Check sheet for the modelled part. Datum: model origin and axes. Units: mm. Face numbers are marked on the shaded views. A direction names the side the tool comes from. Coordinates: 2 decimals unless noted, no trailing zeros. Loops run counter-clockwise (first coordinate to the right, second up) from the corner with the lowest first, then second, coordinate; pieces in that order, holes last. Notation, with made-up numbers: (13.25, 64) -> (67.25, 64) arc R28 cw to (67.25, 89) -> close; hole circle Ø7 at (26.5, -6). An arc over 180 degrees is marked (long way). Use CSV: the item, a comma, the result in double quotes. Start each with the question number.
1. Sectioned sample at D-D, the plane x = 16.25. Record the cut outline in (y, z), and give its area (3 significant figures).
2. Sectioned sample at B-B, the plane z = 12.4. Record the cut outline in (x, y) (3 decimals), and give its area (3 significant figures).
3. Set-up check for the marked faces 4, 5, 6, 7 and 8: record each of +Z, -Z, +X, -X, +Y, -Y from which the full face is reachable in a straight line by a thin tool's end or side.
4. Release check for a two-part mould opening along Z. For the marked faces 1, 2 and 3 record: pulls with the +Z half, pulls with the -Z half, needs draft (parallel to the pull), parting line crosses it, or undercut.
5. Sectioned sample at C-C, the plane z = 4. Record the cut outline in (x, y) (3 decimals).
6. Thickness scan on L1, parallel to X at y = 0.6, z = 12.4; L2, parallel to Z at x = -16.25, y = 8.25; L3, parallel to Z at x = 10.5, y = 4.25 (3 decimals). Record the ranges inside material, lowest first.
7. Gauge pin test, flat ends, axial feed: pin 1 (1 mm diameter, centred on y = 9.5, z = 14, fed in from +X); pin 2 (2 mm diameter, centred on x = 16, z = 17, fed in from -Y); pin 3 (2 mm diameter, centred on x = 2, z = -13, fed in from +Y). Record the tip position at first contact, or that the pin passes through.
8. Sectioned sample at A-A, the plane y = 7. Record the cut outline in (x, z).
```python
from build123d import *

# Parameters (mm, degrees)
SKETCH1_W                      = 40
SKETCH1_H                      = 40
BOSS_EXTRUDE1_DEPTH            = 6.35
SKETCH2_W                      = 11.25
SKETCH2_H                      = 11.25
CUT_EXTRUDE1_DEPTH             = 7.35
SKETCH3_W                      = 14
SKETCH3_H                      = 8.5
CUT_EXTRUDE2_DEPTH             = 2
M2_CLEARANCE_HOLE1_D           = 2.4
SKETCH6_R                      = 2.6
BOSS_EXTRUDE2_DEPTH            = 5
CBORE_FOR_M2_SHCS1_D           = 2.4
CBORE_FOR_M2_SHCS1_CBORE_D     = 4.4
CBORE_FOR_M2_SHCS1_CBORE_DEPTH = 2
SKETCH13_R                     = 2.175
CUT_EXTRUDE4_DEPTH             = 4.2
CHAMFER1_SIZE                  = 2.5


with BuildPart() as part:
    # Sketch1 → Boss-Extrude1 (new body)
    with BuildSketch(Plane(origin=(0, 0, 0), x_dir=(1, 0, 0), z_dir=(0, 1, 0))):
        Rectangle(SKETCH1_W, SKETCH1_H)
    extrude(amount=BOSS_EXTRUDE1_DEPTH)

    # Sketch2 → Cut-Extrude1 (cut, through all)
    with BuildSketch(Plane(origin=(0, 6.35, 0), x_dir=(1, 0, 0), z_dir=(0, 1, 0))):
        Rectangle(SKETCH2_W, SKETCH2_H)
    extrude(amount=-CUT_EXTRUDE1_DEPTH, mode=Mode.SUBTRACT)

    # Sketch3 → Cut-Extrude2 (cut)
    with BuildSketch(Plane(origin=(0, 6.35, 0), x_dir=(1, 0, 0), z_dir=(0, 1, 0))):
        with Locations((0, -9.875)):
            Rectangle(SKETCH3_W, SKETCH3_H)
    extrude(amount=-CUT_EXTRUDE2_DEPTH, mode=Mode.SUBTRACT)

    # M2 Clearance Hole1 (through all)
    with Locations(Plane(origin=(0, 6.35, 0), x_dir=(1, 0, 0), z_dir=(0, 1, 0))):
        with Locations((10.5, 0.1), (10.5, -12.4), (-10.5, -12.4), (-10.5, 0.1)):
            Hole(M2_CLEARANCE_HOLE1_D / 2)

    # Sketch6 → Boss-Extrude2 (add)
    with BuildSketch(Plane(origin=(0, 6.35, 0), x_dir=(1, 0, 0), z_dir=(0, 1, 0))):
        with Locations((-16.25, 16.25)):
            Circle(SKETCH6_R)
        with Locations((16.25, 16.25)):
            Circle(SKETCH6_R)
        with Locations((16.25, -16.25)):
            Circle(SKETCH6_R)
        with Locations((-16.25, -16.25)):
            Circle(SKETCH6_R)
    extrude(amount=BOSS_EXTRUDE2_DEPTH)

    # CBORE for M2 SHCS1 (through all)
    with Locations(Plane.XZ):
        with Locations((-16.25, -16.25), (-16.25, 16.25), (16.25, 16.25), (16.25, -16.25)):
            CounterBoreHole(CBORE_FOR_M2_SHCS1_D / 2, CBORE_FOR_M2_SHCS1_CBORE_D / 2, CBORE_FOR_M2_SHCS1_CBORE_DEPTH)

    # Sketch13 → Cut-Extrude4 (cut)
    with BuildSketch(Plane(origin=(0, 6.35, 0), x_dir=(1, 0, 0), z_dir=(0, 1, 0))):
        with Locations((-10.5, -12.4)):
            Circle(SKETCH13_R)
        with Locations((-10.5, 0.1)):
            Circle(SKETCH13_R)
        with Locations((10.5, -12.4)):
            Circle(SKETCH13_R)
        with Locations((10.5, 0.1)):
            Circle(SKETCH13_R)
    extrude(amount=-CUT_EXTRUDE4_DEPTH, mode=Mode.SUBTRACT)

    # Chamfer1
    chamfer1_edges = [part.edges().sort_by_distance(p)[0] for p in [
        (5.625, 0, 0),
        (0, 0, 5.625),
        (-5.625, 0, 0),
        (0, 0, -5.625),
    ]]
    chamfer(chamfer1_edges, length=CHAMFER1_SIZE)


solid = part.part
```
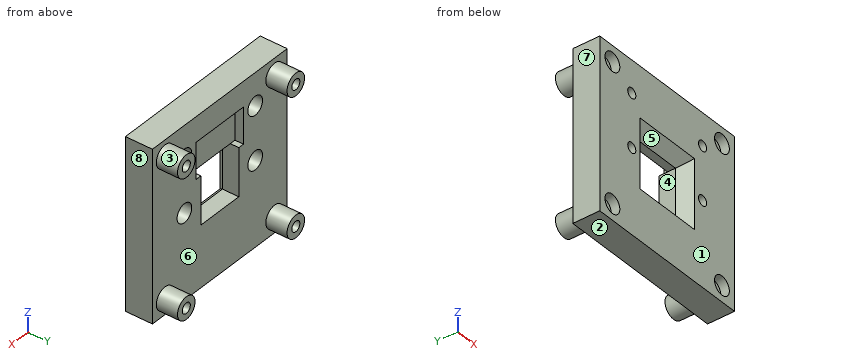
Completed:
1,outline,"(0, -20) -> (6.35, -20) -> (6.35, -18.85) -> (11.35, -18.85) -> (11.35, -17.45) -> (2, -17.45) -> (2, -18.45) -> (0, -18.45) -> close; (0, -14.05) -> (2, -14.05) -> (2, -15.05) -> (11.35, -15.05) -> (11.35, -13.65) -> (6.35, -13.65) -> (6.35, 13.65) -> (11.35, 13.65) -> (11.35, 15.05) -> (2, 15.05) -> (2, 14.05) -> (0, 14.05) -> close; (0, 18.45) -> (2, 18.45) -> (2, 17.45) -> (11.35, 17.45) -> (11.35, 18.85) -> (6.35, 18.85) -> (6.35, 20) -> (0, 20) -> close"
1,area,"244 mm²"
2,outline,"(-20, 0) -> (-11.7, 0) -> (-11.7, 2.15) -> (-12.675, 2.15) -> (-12.675, 6.35) -> (-20, 6.35) -> close; (-9.3, 0) -> (9.3, 0) -> (9.3, 2.15) -> (8.325, 2.15) -> (8.325, 6.35) -> (7, 6.35) -> (7, 4.35) -> (-7, 4.35) -> (-7, 6.35) -> (-8.325, 6.35) -> (-8.325, 2.15) -> (-9.3, 2.15) -> close; (11.7, 0) -> (20, 0) -> (20, 6.35) -> (12.675, 6.35) -> (12.675, 2.15) -> (11.7, 2.15) -> close"
2,area,"179 mm²"
3,face 4,"+Y, -Y"
3,face 5,"-Y"
3,face 6,"+Y"
3,face 7,"+Z, -Z, -X, +Y, -Y"
3,face 8,"+Z, -Z, +X, +Y, -Y"
4,face 1,"needs draft"
4,face 2,"pulls with the -Z half"
4,face 3,"undercut"
5,outline,"(-20, 0) -> (-8.125, 0) -> (-5.625, 2.5) -> (-5.625, 6.35) -> (-20, 6.35) -> close; (5.625, 2.5) -> (8.125, 0) -> (20, 0) -> (20, 6.35) -> (5.625, 6.35) -> close"
6,L1,"-20 to -11.7, -9.3 to 9.3, 11.7 to 20"
6,L2,"-18.85 to -17.45, -15.05 to -13.65, 13.65 to 15.05, 17.45 to 18.85"
6,L3,"-20 to -2.275, 2.075 to 10.225, 14.575 to 20"
7,pin 1,"x = 18.17"
7,pin 2,"y = 2"
7,pin 3,"y = 6.35"
8,outline,"circle Ø5.2 at (-16.25, -16.25); circle Ø5.2 at (-16.25, 16.25); circle Ø5.2 at (16.25, -16.25); circle Ø5.2 at (16.25, 16.25); hole circle Ø2.4 at (-16.25, -16.25); hole circle Ø2.4 at (-16.25, 16.25); hole circle Ø2.4 at (16.25, -16.25); hole circle Ø2.4 at (16.25, 16.25)"
